Input: part model. Units: mm. Frame: model coordinates. A direction names the side the tool comes from. Give positions to 0.01 mm unless a question says otherwise; leave off trailing zeros. Order: outer loops, then holes, each group sorted by start corner. A loop starts at its lowest first (then second) coordinate and runs counter-clockwise, first axis right, second up. Notation, with made-up numbers: (13, 54) -> (39, 54) arc R32 ccw to (39, 81) -> close; hole circle Ø1 at (34.25, -35.5). An arc over 180 degrees is marked (long way). Use a Markdown table: item, result. Add a question column.
from build123d import *

# Parameters (mm, degrees)
DODANIE_WYCI_GNI_CIE1_DEPTH = 6


with BuildPart() as part:
    # Szkic1 → Dodanie-wyciągnięcie1 (new body)
    with BuildSketch(Plane(origin=(0, 0, 0), x_dir=(1, 0, 0), z_dir=(0, 1, 0))):
        with BuildLine():
            Line((-276.493755035, 26.54073282), (-317.199927227, 11.020878293))
            ThreePointArc((-317.199927227, 11.020878293), (-323.470347305, 0), (-317.199927227, -11.020878293))
            Line((-317.199927227, -11.020878293), (-276.493755035, -26.54073282))
            ThreePointArc((-276.493755035, -26.54073282), (-275.267846651, -26.8842258), (-274, -27))
            Line((-274, -27), (274, -27))
            ThreePointArc((274, -27), (276.508698973, -26.535015644), (278.68411058, -25.20183699))
            Line((278.68411058, -25.20183699), (301.877848562, -6.316516345))
            ThreePointArc((301.877848562, -6.316516345), (304.69, 0), (301.877848562, 6.316516345))
            Line((301.877848562, 6.316516345), (278.68411058, 25.20183699))
            ThreePointArc((278.68411058, 25.20183699), (276.508698973, 26.535015644), (274, 27))
            Line((274, 27), (-274, 27))
            ThreePointArc((-274, 27), (-275.267846651, 26.8842258), (-276.493755035, 26.54073282))
        make_face()
        with BuildLine():
            ThreePointArc((-318.031465247, 9.633625156), (-322.786422983, 0), (-318.031465247, -9.633625156))
            Line((-318.031465247, -9.633625156), (-276.137504316, -25.606342417))
            ThreePointArc((-276.137504316, -25.606342417), (-275.086725701, -25.900764972), (-274, -26))
            Line((-274, -26), (274, -26))
            ThreePointArc((274, -26), (276.150313405, -25.60144198), (278.014951926, -24.45871742))
            Line((278.014951926, -24.45871742), (301.208689908, -5.573396775))
            ThreePointArc((301.208689908, -5.573396775), (303.69, 0), (301.208689908, 5.573396775))
            Line((301.208689908, 5.573396775), (278.014951926, 24.45871742))
            ThreePointArc((278.014951926, 24.45871742), (276.150313405, 25.60144198), (274, 26))
            Line((274, 26), (-274, 26))
            ThreePointArc((-274, 26), (-275.086725701, 25.900764972), (-276.137504316, 25.606342417))
            Line((-276.137504316, 25.606342417), (-318.031465247, 9.633625156))
        make_face(mode=Mode.SUBTRACT)
    extrude(amount=DODANIE_WYCI_GNI_CIE1_DEPTH)


solid = part.part
Q1. First-contact query: pin 1 (10 mm diameter, centred on x = -130.5, z = 21.5, fed in from +Y); pin 2 (1.5 mm diameter, centred on y = 3.5, z = -15, fed in from +X). Flat tips, straight axial feed; report the tip coordinate or a pass-through.
Q2. Section query B-B (x = 177). Return loops of the section in (y, z).
Q3. Draft query along X for faces 3 (the flat face through (289.774, 2.958, -14.884)), 4 (the flat face through (290.12, 2.96, 15.89)), 5 (the flat face through (-297.132, 2.958, 18.672)), 6 (the flat face through (289.45, 2.96, 15.15)). Return one class per face: +X half, -X half, draft (parallel to the pull), parting line (faces both ways), or undercut.
Q4. Access query for faces 1 (the flat face through (-296.56, 2.96, -18.89)), 2 (the flat face through (-296.791, 2.958, -17.732)). Directions: +Z, -Z, +X, -X, +Y, -Y. A direction counts if a zero-diameter tool reaches every point of the face in a straight line with its end or side. Return the directions, or none.
Q5. Ray query, line 1 (Z direction, x = 68.5, y = 4.75); line 2 (X direction, y = 1, z = 0); line 3 (X direction, y = 5.2, z = -1). Return the intervals inside material, ascending.
Q6. Section query A-A (y = 4.55). Return loops of the section in (x, z).
Solution:
| question | item | result |
|---|---|---|
| 1 | pin 1 | stops at y = 6 |
| 1 | pin 2 | stops at x = 292.13 |
| 2 | outline | (0, -27) -> (6, -27) -> (6, -26) -> (0, -26) -> close; (0, 26) -> (6, 26) -> (6, 27) -> (0, 27) -> close |
| 3 | face 3 | undercut |
| 3 | face 4 | +X half |
| 3 | face 5 | -X half |
| 3 | face 6 | undercut |
| 4 | face 1 | -Z, -X, +Y, -Y |
| 4 | face 2 | +Y, -Y |
| 5 | line 1 | z = -27 to -26, 26 to 27 |
| 5 | line 2 | x = -323.47 to -322.79, 303.69 to 304.69 |
| 5 | line 3 | x = -323.43 to -322.75, 303.62 to 304.63 |
| 6 | outline | (-317.2, -11.02) -> (-276.49, -26.54) arc R7 ccw to (-274, -27) -> (274, -27) arc R7 ccw to (278.68, -25.2) -> (301.88, -6.32) arc R8.5 ccw to (301.88, 6.32) -> (278.68, 25.2) arc R7 ccw to (274, 27) -> (-274, 27) arc R7 ccw to (-276.49, 26.54) -> (-317.2, 11.02) arc R12.82 ccw to start; hole (-318.03, -9.63) -> (-276.14, -25.61) arc R6 ccw to (-274, -26) -> (274, -26) arc R6 ccw to (278.01, -24.46) -> (301.21, -5.57) arc R7.5 ccw to (301.21, 5.57) -> (278.01, 24.46) arc R6 ccw to (274, 26) -> (-274, 26) arc R6 ccw to (-276.14, 25.61) -> (-318.03, 9.63) arc R12.14 ccw to start |
